```python
from build123d import *

# Parameters (mm, degrees)
F0_R     = 2.55
F1_DEPTH = 6.35
F2_R     = 5
F3_R     = 5


with BuildPart() as f1:
    # F0 (on Top) → F1 (new body)
    with BuildSketch(Plane.XY):
        Polygon((0, 101.5), (0, 0), (127, 0), (127, 54), (100, 54), (79.5, 74.5), (79.5, 101.5), align=None)
        with BuildLine():
            ThreePointArc((36, 64.95), (34.5504310986, 68.4495689014), (38.05, 67))
            Line((38.05, 67), (73.95, 67))
            ThreePointArc((73.95, 67), (76, 69.05), (78.05, 67))
            ThreePointArc((78.05, 67), (77.4495689014, 65.5504310986), (76, 64.95))
            Line((76, 64.95), (76, 52.25))
            ThreePointArc((76, 52.25), (79.7123106012, 50.7123106012), (81.25, 47))
            ThreePointArc((81.25, 47), (79.7123106012, 43.2876893988), (76, 41.75))
            Line((76, 41.75), (76, 29.05))
            ThreePointArc((76, 29.05), (77.4495689014, 28.4495689014), (78.05, 27))
            ThreePointArc((78.05, 27), (76, 24.95), (73.95, 27))
            Line((73.95, 27), (38.05, 27))
            ThreePointArc((38.05, 27), (34.5504310986, 25.5504310986), (36, 29.05))
            Line((36, 29.05), (36, 64.95))
        make_face(mode=Mode.SUBTRACT)
        with Locations((116, 20.75)):
            Circle(F0_R, mode=Mode.SUBTRACT)
        with Locations((116, 45.75)):
            Circle(F0_R, mode=Mode.SUBTRACT)
        with Locations((10, 91)):
            Circle(F0_R, mode=Mode.SUBTRACT)
        with Locations((50.25, 91)):
            Circle(F0_R, mode=Mode.SUBTRACT)
        with BuildLine():
            Line((73.95, 67), (38.05, 67))
            ThreePointArc((38.05, 67), (37.4495689014, 65.5504310986), (36, 64.95))
            Line((36, 64.95), (36, 29.05))
            ThreePointArc((36, 29.05), (37.4495689014, 28.4495689014), (38.05, 27))
            Line((38.05, 27), (73.95, 27))
            ThreePointArc((73.95, 27), (74.5504310986, 28.4495689014), (76, 29.05))
            Line((76, 29.05), (76, 41.75))
            ThreePointArc((76, 41.75), (70.75, 47), (76, 52.25))
            Line((76, 52.25), (76, 64.95))
            ThreePointArc((76, 64.95), (74.5504310986, 65.5504310986), (73.95, 67))
        make_face()
    extrude(amount=F1_DEPTH)

    # F2
    f2_edges = [f1.edges().sort_by_distance(p)[0] for p in [
        (79.5, 74.5, 3.175),
        (100, 54, 3.175),
    ]]
    fillet(f2_edges, radius=F2_R)

    # F3
    f3_edges = [f1.edges().sort_by_distance(p)[0] for p in [
        (0, 101.5, 3.175),
        (79.5, 101.5, 3.175),
        (127, 54, 3.175),
        (127, 0, 3.175),
        (0, 0, 3.175),
    ]]
    fillet(f3_edges, radius=F3_R)


solid = f1.part
```
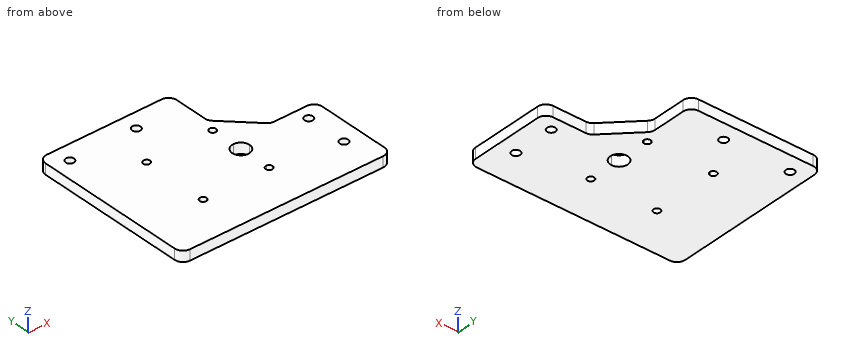
Geometry: final body of the model. Coordinates: model frame, mm. Round coordinates to 2 decimals unless told otherwise and drop trailing zeros. Write each loop counter-clockwise with the first axis right and the second up, starting at its lowest first coordinate (ties: lowest second). Pieces come first, ordered by that corner, then holes. Notation, with made-up numbers: (60, 51) -> (114, 51) arc R34 cw to (114, 85) -> close; hole circle Ø7 at (5.25, 87.25). An arc over 180 degrees is marked (long way). Use CSV: the item, a comma, the result in double quotes. Start each with the question number.
Q1. First-contact query: pin 1 Ø8 at (x, y) = (10, 91) entering from -Z; pin 2 Ø2 at (y, z) = (78, 2.5) entering from +X; pin 3 Ø3 at (x, z) = (102, 1) entering from +Y; pin 4 Ø3 at (x, z) = (114.5, 2.5) entering from +Y. Flat tips, straight axial feed; report the tip coordinate or a pass-through.
Q2. Section B-B (y = 20.75). Return loops of the section in (x, z).
Q3. Section A-A (x = 10). Return loops of the section in (y, z), plus the area to 3 significant figures.
Q4. Section C-C (z = 1.25). Give the number of separate pieces and of enclosed holes in the cut face, plus the area to 3 significant figures.
Q5. Line query: L1, parallel to Y at x = 116, z = 2.5; L2, parallel to Y at x = 36, z = 2.75; L3, parallel to X at y = 45.5, z = 4. Output: solid intervals per line, ascending.
Q6. Section D-D (y = 91). Return loops of the section in (x, z), plus the area to 3 significant figures.
Result sheet:
1,pin 1,"z = 0"
1,pin 2,"x = 79.5"
1,pin 3,"y = 54.25"
1,pin 4,"y = 54"
2,outline,"(0, 0) -> (113.45, 0) -> (113.45, 6.35) -> (0, 6.35) -> close; (118.55, 0) -> (127, 0) -> (127, 6.35) -> (118.55, 6.35) -> close"
3,outline,"(0, 0) -> (88.45, 0) -> (88.45, 6.35) -> (0, 6.35) -> close; (93.55, 0) -> (101.5, 0) -> (101.5, 6.35) -> (93.55, 6.35) -> close"
3,area,"612 mm²"
4,separate pieces,"1"
4,enclosed holes,"9"
4,area,"10,600 mm²"
5,L1,"0 to 18.2, 23.3 to 43.2, 48.3 to 54"
5,L2,"0 to 24.95, 29.05 to 64.95, 69.05 to 101.5"
5,L3,"0 to 70.97, 81.03 to 113.46, 118.54 to 127"
6,outline,"(0, 0) -> (7.45, 0) -> (7.45, 6.35) -> (0, 6.35) -> close; (12.55, 0) -> (47.7, 0) -> (47.7, 6.35) -> (12.55, 6.35) -> close; (52.8, 0) -> (79.5, 0) -> (79.5, 6.35) -> (52.8, 6.35) -> close"
6,area,"440 mm²"
